For this review, take the finished solid that the model builds, in its own axes (mm). Face numbers are marked on the shaded views. A direction names the side the tool comes from. Round coordinates to 2 decimals unless told otherwise and drop trailing zeros. Write each loop counter-clockwise with the first axis right and the second up, starting at its lowest first coordinate (ties: lowest second). Pieces come first, ordered by that corner, then holes. Notation, with made-up numbers: (10.25, 82.5) -> (25.25, 82.5) arc R18 cw to (25.25, 97.5) -> close; hole circle Ø2 at (-31.5, 46). An arc over 180 degrees is marked (long way). Write each question's results on one line, items separated by ' | '. Start each with the question number.
Item 1: Add section B-B (x = 0). State the section outline as (y, z) points.
Item 2: To check wall thickness, follow line 1 along Y through (x, z) = (0, 4); line 2 along Z through (x, y) = (1.75, -0.25); line 3 along X through (y, z) = (-0.7, 9). State the ranges of each line that lie inside material, in increasing order.
Item 3: The part is to be moulded in two halves that separate along Y. For the marked faces 1, 2 and 3, say which applies: +Y half, -Y half, draft (parallel to the pull), parting line (faces both ways), or undercut.
Item 4: Tool access review of the marked faces 4 and 5: name each direction out of +Z, -Z, +X, -X, +Y, -Y from which nothing blocks a thin tool from reaching the whole face with its end or side.
Item 5: Add section D-D (y = 1.75). State the section outline as (x, z) points.
Item 6: Add section C-C (z = -0.25). State the section outline as (x, y) points, plus the area to 3 significant figures.
Item 7: Add section A-A (z = 2.75). State the section outline as (x, y) points.
Item 8: Clearance check with a flat-ended pin moving along its axis: pin 1 (2 mm diameter, centred on y = -0.5, z = 7, fed in from +X). State where the tip first meets the part, or that it passes through.
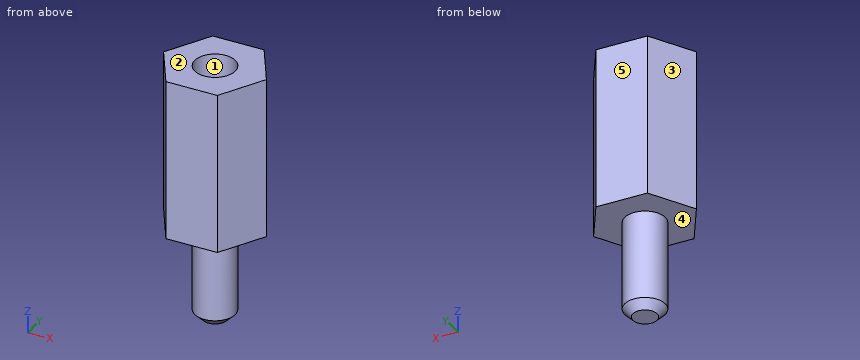
Autodesk Inventor part; units mm, degrees
ref_plane "YZ Plane" through (0, 0, 0) normal (1, 0, 0) x (0, 1, 0)
ref_plane "XZ Plane" through (0, 0, 0) normal (0, 1, 0) x (-1, 0, 0)
ref_plane "XY Plane" through (0, 0, 0) normal (0, 0, 1) x (1, 0, 0)
sketch "Skizze1" plane through (0, 0, 0) normal (0, 0, 1) x (1, 0, 0)
  line L0 (1.5877, 2.75) -> (3.1754, 0)
  line L1 (3.1754, 0) -> (1.5877, -2.75)
  line L2 (1.5877, -2.75) -> (-1.5877, -2.75)
  line L3 (-1.5877, -2.75) -> (-3.1754, 0)
  line L4 (-3.1754, 0) -> (-1.5877, 2.75)
  line L5 (-1.5877, 2.75) -> (1.5877, 2.75)
  circle A0 centre (0, 0) radius 1.25
  circle A1 centre (0, 0) radius 1.5
  point P0 (0, -2.75)
  dimension "d0" = 5.5
  dimension "d1" = 2.5
  dimension "d2" = 3
extrude "Extrusion1" add sketch "Skizze1" along normal blind 10 contours L0 L1 L2 L3 L4 L5 | A1
extrude "Extrusion2" add sketch "Skizze1" along normal blind 2 contours A0
extrude "Extrusion3" add sketch "Skizze1" against normal blind 6 contours A0
chamfer "Fase1" distance 0.5 angle 45 1 edges at (-1.25, 0, -6)
properties part number "M3x10x6 Standoff" material "Edelstahl"
Responses:
1) outline: (-2.75, 0) -> (-1.25, 0) -> (-1.25, -5.5) -> (-0.75, -6) -> (0.75, -6) -> (1.25, -5.5) -> (1.25, 0) -> (2.75, 0) -> (2.75, 10) -> (1.25, 10) -> (1.25, 2) -> (-1.25, 2) -> (-1.25, 10) -> (-2.75, 10) -> close
2) line 1: y = -2.75 to -1.25, 1.25 to 2.75 | line 2: z = 0 to 10 | line 3: x = -2.77 to -1.04, 1.04 to 2.77
3) face 1: undercut | face 2: draft | face 3: +Y half
4) face 4: -Z | face 5: +Z, -Z, +X, -X, +Y
5) outline: (-2.17, 0) -> (2.17, 0) -> (2.17, 10) -> (-2.17, 10) -> close
6) outline: circle Ø2.5 at (0, 0) | area: 4.91 mm^2
7) outline: (-3.18, 0) -> (-1.59, -2.75) -> (1.59, -2.75) -> (3.18, 0) -> (1.59, 2.75) -> (-1.59, 2.75) -> close; hole circle Ø2.5 at (0, 0)
8) pin 1: stops at x = 3.18
